Can you work these out from the model? Positions are in its coordinate system, mm. A direction names the side the tool comes from. Coordinates: 2 decimals unless noted, no trailing zeros. Order: outer loops, then holes, each group sorted by start corner. A loop starts at its lowest first (then second) coordinate and runs counter-clockwise, first axis right, second up. Notation, with made-up numbers: (48.25, -36.75) - (89.25, -36.75) arc R19 cw to (89.25, -15.75) - close; hole circle Ø8 at (-40, 15.25). An arc over 180 degrees is marked (long way). Use a Markdown table: item, result. Add a question column.
(1) On a 3-axis mill with a long thin cutter (end or side, diameter ignored), from which of +Z, -Z, +X, -X, +Y, -Y can I reach the whole of each face in a straight line? I mean faces 5 (the cylindrical face through (-14.985, 0.66, 9.86)), 6 (the flat face through (3, -10, 20)). Say none if no direction works.
(2) We'd pull the mould along X, two halves only. Please class faces 1 (the flat face through (3, -10, 0)), 2 (the cylindrical face through (2.17, 9.76, 24.93)), 3 (the flat face through (0, -2, 10)), 4 (the cylindrical face through (-2.17, -9.76, 5.07)): pulls with the +X half, pulls with the -X half, needs draft (parallel to the pull), parting line crosses it, or undercut.
(3) For pin 1 Ø4 at (x, z) = (-8.5, 3.5) entering from +Y; pin 2 Ø0.6 at (x, z) = (4, 11.5) entering from +Y; pin 3 Ø0.8 at (x, z) = (-1.5, 11) entering from -Y, each with a flat end and sliding along its axis, tell me the tip position at first contact or that it passes through.
(4) I want a section at C-C (x = -9.5). List the corners of the cut face in (y, z) for me.
(5) I want a section at D-D (y = -12.25). List the corners of the cut face in (x, z) for me, and give its area (3 significant figures).
(6) I want a section at A-A (z = 14.5). List the corners of the cut face in (x, y) for me.
(7) I want a section at B-B (x = 6). List the corners of the cut face in (y, z) for me.
(8) If I drill on L1, parallel to Y at x = 0, z = 5; L2, parallel to Y at x = 0, z = 23.25; L3, parallel to Z at x = -12.5, y = -8, over which ranges is the centre line in solid material (lowest first)? Write a range as [from, to].
```python
from build123d import *

# Parameters (mm, degrees)
SKETCH1_R                  = 15
BOSS_EXTRUDE1_DEPTH        = 10
SKETCH2_R                  = 10
CUT_EXTRUDE1_DEPTH         = 20
SKETCH3_R                  = 15
BOSS_EXTRUDE2_DEPTH        = 10
SKETCH5_R                  = 10
CUT_EXTRUDE3_DEPTH         = 8
SKETCH8_W                  = 0.75
SKETCH8_H                  = 0.75
CUT_EXTRUDE5_DEPTH         = 2
FILL_START                 = -1.125
FILL_PATTERN2_OUTLINE_W    = 0.75
FILL_PATTERN2_OUTLINE_H    = 2
FILL_PATTERN2_DEPTH        = 0.75
FILL_START_2               = 0.375
FILL_PATTERN2_2_OUTLINE_W  = 0.75
FILL_PATTERN2_2_OUTLINE_H  = 2
FILL_PATTERN2_2_DEPTH      = 0.75
FILL_START_3               = -3.375
FILL_PATTERN2_3_OUTLINE_W  = 0.75
FILL_PATTERN2_3_OUTLINE_H  = 2
FILL_PATTERN2_3_DEPTH      = 0.75
FILL_START_4               = -1.875
FILL_PATTERN2_4_OUTLINE_W  = 0.75
FILL_PATTERN2_4_OUTLINE_H  = 2
FILL_PATTERN2_4_DEPTH      = 0.75
FILL_START_5               = 1.125
FILL_PATTERN2_5_OUTLINE_W  = 0.75
FILL_PATTERN2_5_OUTLINE_H  = 2
FILL_PATTERN2_5_DEPTH      = 0.75
FILL_START_6               = 2.625
FILL_PATTERN2_6_OUTLINE_W  = 0.75
FILL_PATTERN2_6_OUTLINE_H  = 2
FILL_PATTERN2_6_DEPTH      = 0.75
FILL_START_7               = -4.125
FILL_PATTERN2_7_OUTLINE_W  = 0.75
FILL_PATTERN2_7_OUTLINE_H  = 2
FILL_PATTERN2_7_DEPTH      = 0.75
FILL_START_8               = -2.625
FILL_PATTERN2_8_OUTLINE_W  = 0.75
FILL_PATTERN2_8_OUTLINE_H  = 2
FILL_PATTERN2_8_DEPTH      = 0.75
FILL_START_9               = -0.375
FILL_PATTERN2_9_OUTLINE_W  = 0.75
FILL_PATTERN2_9_OUTLINE_H  = 2
FILL_PATTERN2_9_DEPTH      = 0.75
FILL_START_10              = 1.875
FILL_PATTERN2_10_OUTLINE_W = 0.75
FILL_PATTERN2_10_OUTLINE_H = 2
FILL_PATTERN2_10_DEPTH     = 0.75
FILL_START_11              = 3.375
FILL_PATTERN2_11_OUTLINE_W = 0.75
FILL_PATTERN2_11_OUTLINE_H = 2
FILL_PATTERN2_11_DEPTH     = 0.75
SKETCH12_W                 = 18
SKETCH12_H                 = 5


# Read off the part's stored shape, not the designer's step: Fill Pattern2
with BuildPart() as part:
    # Sketch1 → Boss-Extrude1 (new body)
    with BuildSketch(Plane.XY):
        Circle(SKETCH1_R)
    extrude(amount=BOSS_EXTRUDE1_DEPTH)

    # Sketch2 → Cut-Extrude1 (cut)
    with BuildSketch(Plane.XY.offset(10)):
        Circle(SKETCH2_R)
    extrude(amount=-CUT_EXTRUDE1_DEPTH, mode=Mode.SUBTRACT)

    # Sketch3 → Boss-Extrude2 (add)
    with BuildSketch(Plane.XY.offset(10)):
        Circle(SKETCH3_R)
    extrude(amount=BOSS_EXTRUDE2_DEPTH)

    # Sketch5 → Cut-Extrude3 (cut)
    with BuildSketch(Plane.XY.offset(20)):
        Circle(SKETCH5_R)
    extrude(amount=-CUT_EXTRUDE3_DEPTH, mode=Mode.SUBTRACT)

    # Sketch8 → Cut-Extrude5 (cut)
    with BuildSketch(Plane(origin=(0, 0, 10), x_dir=(-1, 0, 0), z_dir=(0, 0, -1))):
        Rectangle(SKETCH8_W, SKETCH8_H)
    extrude(amount=-CUT_EXTRUDE5_DEPTH, mode=Mode.SUBTRACT)

    # Fill Pattern2 outline → Fill Pattern2 (cut)
    with BuildSketch(Plane.YZ.offset(FILL_START)):
        with Locations((-1.299038106, 11)):
            Rectangle(FILL_PATTERN2_OUTLINE_W, FILL_PATTERN2_OUTLINE_H)
        with Locations((1.299038106, 11)):
            Rectangle(FILL_PATTERN2_OUTLINE_W, FILL_PATTERN2_OUTLINE_H)
        with Locations((-3.897114317, 11)):
            Rectangle(FILL_PATTERN2_OUTLINE_W, FILL_PATTERN2_OUTLINE_H)
        with Locations((3.897114317, 11)):
            Rectangle(FILL_PATTERN2_OUTLINE_W, FILL_PATTERN2_OUTLINE_H)
    extrude(amount=FILL_PATTERN2_DEPTH, mode=Mode.SUBTRACT)

    # Fill Pattern2 2 outline → Fill Pattern2 2 (cut)
    with BuildSketch(Plane.YZ.offset(FILL_START_2)):
        with Locations((-1.299038106, 11)):
            Rectangle(FILL_PATTERN2_2_OUTLINE_W, FILL_PATTERN2_2_OUTLINE_H)
        with Locations((1.299038106, 11)):
            Rectangle(FILL_PATTERN2_2_OUTLINE_W, FILL_PATTERN2_2_OUTLINE_H)
        with Locations((-3.897114317, 11)):
            Rectangle(FILL_PATTERN2_2_OUTLINE_W, FILL_PATTERN2_2_OUTLINE_H)
        with Locations((3.897114317, 11)):
            Rectangle(FILL_PATTERN2_2_OUTLINE_W, FILL_PATTERN2_2_OUTLINE_H)
    extrude(amount=FILL_PATTERN2_2_DEPTH, mode=Mode.SUBTRACT)

    # Fill Pattern2 3 outline → Fill Pattern2 3 (cut)
    with BuildSketch(Plane.YZ.offset(FILL_START_3)):
        with Locations((0, 11)):
            Rectangle(FILL_PATTERN2_3_OUTLINE_W, FILL_PATTERN2_3_OUTLINE_H)
        with Locations((-2.598076211, 11)):
            Rectangle(FILL_PATTERN2_3_OUTLINE_W, FILL_PATTERN2_3_OUTLINE_H)
        with Locations((2.598076211, 11)):
            Rectangle(FILL_PATTERN2_3_OUTLINE_W, FILL_PATTERN2_3_OUTLINE_H)
    extrude(amount=FILL_PATTERN2_3_DEPTH, mode=Mode.SUBTRACT)

    # Fill Pattern2 4 outline → Fill Pattern2 4 (cut)
    with BuildSketch(Plane.YZ.offset(FILL_START_4)):
        with Locations((0, 11)):
            Rectangle(FILL_PATTERN2_4_OUTLINE_W, FILL_PATTERN2_4_OUTLINE_H)
        with Locations((-2.598076211, 11)):
            Rectangle(FILL_PATTERN2_4_OUTLINE_W, FILL_PATTERN2_4_OUTLINE_H)
        with Locations((2.598076211, 11)):
            Rectangle(FILL_PATTERN2_4_OUTLINE_W, FILL_PATTERN2_4_OUTLINE_H)
    extrude(amount=FILL_PATTERN2_4_DEPTH, mode=Mode.SUBTRACT)

    # Fill Pattern2 5 outline → Fill Pattern2 5 (cut)
    with BuildSketch(Plane.YZ.offset(FILL_START_5)):
        with Locations((0, 11)):
            Rectangle(FILL_PATTERN2_5_OUTLINE_W, FILL_PATTERN2_5_OUTLINE_H)
        with Locations((-2.598076211, 11)):
            Rectangle(FILL_PATTERN2_5_OUTLINE_W, FILL_PATTERN2_5_OUTLINE_H)
        with Locations((2.598076211, 11)):
            Rectangle(FILL_PATTERN2_5_OUTLINE_W, FILL_PATTERN2_5_OUTLINE_H)
    extrude(amount=FILL_PATTERN2_5_DEPTH, mode=Mode.SUBTRACT)

    # Fill Pattern2 6 outline → Fill Pattern2 6 (cut)
    with BuildSketch(Plane.YZ.offset(FILL_START_6)):
        with Locations((0, 11)):
            Rectangle(FILL_PATTERN2_6_OUTLINE_W, FILL_PATTERN2_6_OUTLINE_H)
        with Locations((-2.598076211, 11)):
            Rectangle(FILL_PATTERN2_6_OUTLINE_W, FILL_PATTERN2_6_OUTLINE_H)
        with Locations((2.598076211, 11)):
            Rectangle(FILL_PATTERN2_6_OUTLINE_W, FILL_PATTERN2_6_OUTLINE_H)
    extrude(amount=FILL_PATTERN2_6_DEPTH, mode=Mode.SUBTRACT)

    # Fill Pattern2 7 outline → Fill Pattern2 7 (cut)
    with BuildSketch(Plane.YZ.offset(FILL_START_7)):
        with Locations((-1.299038106, 11)):
            Rectangle(FILL_PATTERN2_7_OUTLINE_W, FILL_PATTERN2_7_OUTLINE_H)
        with Locations((1.299038106, 11)):
            Rectangle(FILL_PATTERN2_7_OUTLINE_W, FILL_PATTERN2_7_OUTLINE_H)
    extrude(amount=FILL_PATTERN2_7_DEPTH, mode=Mode.SUBTRACT)

    # Fill Pattern2 8 outline → Fill Pattern2 8 (cut)
    with BuildSketch(Plane.YZ.offset(FILL_START_8)):
        with Locations((-1.299038106, 11)):
            Rectangle(FILL_PATTERN2_8_OUTLINE_W, FILL_PATTERN2_8_OUTLINE_H)
        with Locations((1.299038106, 11)):
            Rectangle(FILL_PATTERN2_8_OUTLINE_W, FILL_PATTERN2_8_OUTLINE_H)
    extrude(amount=FILL_PATTERN2_8_DEPTH, mode=Mode.SUBTRACT)

    # Fill Pattern2 9 outline → Fill Pattern2 9 (cut)
    with BuildSketch(Plane.YZ.offset(FILL_START_9)):
        with Locations((-2.598076211, 11)):
            Rectangle(FILL_PATTERN2_9_OUTLINE_W, FILL_PATTERN2_9_OUTLINE_H)
        with Locations((2.598076211, 11)):
            Rectangle(FILL_PATTERN2_9_OUTLINE_W, FILL_PATTERN2_9_OUTLINE_H)
    extrude(amount=FILL_PATTERN2_9_DEPTH, mode=Mode.SUBTRACT)

    # Fill Pattern2 10 outline → Fill Pattern2 10 (cut)
    with BuildSketch(Plane.YZ.offset(FILL_START_10)):
        with Locations((-1.299038106, 11)):
            Rectangle(FILL_PATTERN2_10_OUTLINE_W, FILL_PATTERN2_10_OUTLINE_H)
        with Locations((1.299038106, 11)):
            Rectangle(FILL_PATTERN2_10_OUTLINE_W, FILL_PATTERN2_10_OUTLINE_H)
    extrude(amount=FILL_PATTERN2_10_DEPTH, mode=Mode.SUBTRACT)

    # Fill Pattern2 11 outline → Fill Pattern2 11 (cut)
    with BuildSketch(Plane.YZ.offset(FILL_START_11)):
        with Locations((-1.299038106, 11)):
            Rectangle(FILL_PATTERN2_11_OUTLINE_W, FILL_PATTERN2_11_OUTLINE_H)
        with Locations((1.299038106, 11)):
            Rectangle(FILL_PATTERN2_11_OUTLINE_W, FILL_PATTERN2_11_OUTLINE_H)
    extrude(amount=FILL_PATTERN2_11_DEPTH, mode=Mode.SUBTRACT)

    # Sketch12 → Revolve2 (revolve)
    with BuildSketch(Plane(origin=(0, 0, 0), x_dir=(0, 0, -1), z_dir=(1, 0, 0)), mode=Mode.PRIVATE) as revolve2_sk:
        with Locations((-21, -7.5)):
            Rectangle(SKETCH12_W, SKETCH12_H)
    revolve(revolve2_sk.sketch.rotate(Axis((0, 0, 0), (0, 0, 1)), 270), axis=Axis((0, 0, 0), (0, 0, 1)))


solid = part.part
```
Answers follow:
| question | item | result |
|---|---|---|
| 1 | face 5 | +Z, -Z |
| 1 | face 6 | +Z |
| 2 | face 1 | needs draft |
| 2 | face 2 | parting line crosses it |
| 2 | face 3 | undercut |
| 2 | face 4 | undercut |
| 3 | pin 1 | stops at y = 13.52 |
| 3 | pin 2 | stops at y = 14.54 |
| 3 | pin 3 | stops at y = -14.96 |
| 4 | outline | (-11.61, 0) - (-3.12, 0) - (-3.12, 10) - (3.12, 10) - (3.12, 0) - (11.61, 0) - (11.61, 20) - (3.12, 20) - (3.12, 30) - (-3.12, 30) - (-3.12, 20) - (-11.61, 20) - close |
| 5 | outline | (-8.66, 0) - (8.66, 0) - (8.66, 20) - (-8.66, 20) - close |
| 5 | area | 346 mm² |
| 6 | outline | circle Ø30 at (0, 0); hole circle Ø10 at (0, 0) |
| 7 | outline | (-13.75, 0) - (-8, 0) - (-8, 10) - (8, 10) - (8, 0) - (13.75, 0) - (13.75, 20) - (8, 20) - (8, 30) - (-8, 30) - (-8, 20) - (-13.75, 20) - close |
| 8 | L1 | y = [-15, -10], [10, 15] |
| 8 | L2 | y = [-10, -5], [5, 10] |
| 8 | L3 | z = [0, 20] |
